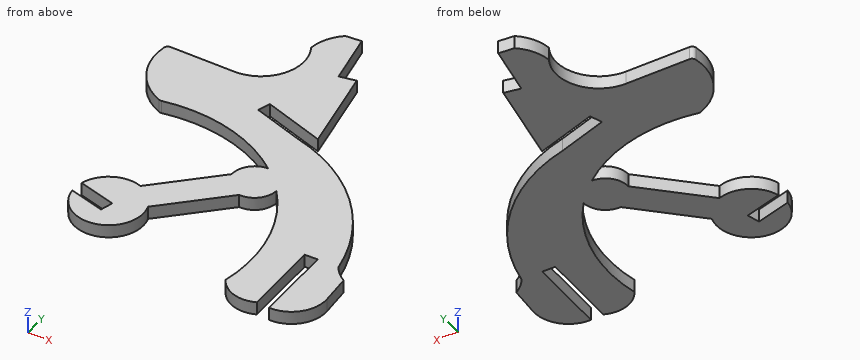
from build123d import *

# Parameters (mm, degrees)
BASE_EXTRUDE_DEPTH = 3


with BuildPart() as part:
    # Sketch1 → Base-Extrude (new body)
    with BuildSketch(Plane.XY):
        with BuildLine():
            Line((293.989820862, 734.197583092), (308.230093844, 729.586709902))
            Line((308.230093844, 729.586709902), (304.237578804, 749.960041406))
            Line((304.237578804, 749.960041406), (300.46187699, 749.205127022))
            Line((300.46187699, 749.205127022), (298.014696403, 761.444692703))
            Line((298.014696403, 761.444692703), (294.380010045, 761.126528526))
            ThreePointArc((294.380010045, 761.126528526), (291.873265467, 758.05762637), (290.76086587, 754.254404584))
            ThreePointArc((290.76086587, 754.254404584), (290.815065416, 744.34095117), (282.238682163, 739.368512483))
            Line((282.238682163, 739.368512483), (267.309755895, 739.368512483))
            ThreePointArc((267.309755895, 739.368512483), (266.660852695, 739.129383455), (266.322292677, 738.526361756))
            ThreePointArc((266.322292677, 738.526361756), (267.945922187, 729.535060668), (274.828113717, 723.525476008))
            ThreePointArc((274.828113717, 723.525476008), (275.107735881, 723.458131465), (275.394960471, 723.473160687))
            ThreePointArc((275.394960471, 723.473160687), (291.10707298, 723.128304911), (305.196249522, 716.165223024))
            ThreePointArc((305.196249522, 716.165223024), (301.525955586, 714.485747009), (300.152427977, 710.690339367))
            Line((300.152427977, 710.690339367), (287.135003329, 697.672914719))
            ThreePointArc((287.135003329, 697.672914719), (280.788235339, 697.185935894), (276.80604128, 692.2199775))
            Line((276.80604128, 692.2199775), (285.544339655, 689.832249216))
            Line((285.544339655, 689.832249216), (284.7535812, 686.938339057))
            Line((284.7535812, 686.938339057), (276.578441435, 689.172182037))
            ThreePointArc((276.578441435, 689.172182037), (286.308923255, 682.31315648), (292.084750798, 692.72316725))
            Line((292.084750798, 692.72316725), (305.102175446, 705.740591898))
            ThreePointArc((305.102175446, 705.740591898), (308.909028424, 707.124695347), (310.57796115, 710.815567264))
            ThreePointArc((310.57796115, 710.815567264), (317.662772954, 696.617074851), (318.003459515, 680.752785464))
            ThreePointArc((318.003459515, 680.752785464), (322.040475508, 677.537424223), (327.190781226, 677.869684733))
            Line((327.190781226, 677.869684733), (326.648810255, 696.184005937))
            Line((326.648810255, 696.184005937), (329.647496764, 696.272745292))
            Line((329.647496764, 696.272745292), (330.19785257, 677.675083141))
            ThreePointArc((330.19785257, 677.675083141), (336.159788883, 680.193967384), (338.280950791, 686.308714689))
            Line((338.280950791, 686.308714689), (337.692715429, 693.239584422))
            ThreePointArc((337.692715429, 693.239584422), (335.883457798, 694.612751583), (334.465786033, 696.387352382))
            ThreePointArc((334.465786033, 696.387352382), (324.143791375, 716.336225522), (304.697858302, 727.577079591))
            Line((304.697858302, 727.577079591), (293.065685578, 731.343473215))
            Line((293.065685578, 731.343473215), (293.989820862, 734.197583092))
        make_face()
    extrude(amount=BASE_EXTRUDE_DEPTH)


solid = part.part
The listing builds one solid part. Answer for the finished solid, in the listing's coordinates (mm). Coordinates: 2 decimals unless noted, no trailing zeros. Order: outer loops, then holes, each group sorted by start corner. A loop starts at its lowest first (then second) coordinate and runs counter-clockwise, first axis right, second up.
Q1. Consider line 1 (Y direction, x = 281, z = 2.85); line 2 (Y direction, x = 278, z = 0.4); line 3 (X direction, y = 693, z = 2.8). Determine where each line is inside the solid, lowest interval first.
Q2. A cutting plane is placed at B-B, the plane y = 753. Write down the section's boundary in (x, z), and give its area (3 significant figures).
Q3. A cutting plane is placed at C-C, the plane x = 315.5. Write down the section's boundary in (y, z).
Q4. Given P1, Ø1, axis at y = 749, z = 1.5, coming from the +X side, flat-ended and moving along its own axis, determine where the tip first touches the part or whether it passes through.
Answers follow:
1. line 1: y = 682.93 to 687.96, 691.07 to 697.29, 724.14 to 739.37
1. line 2: y = 685.48 to 688.78, 691.89 to 694.74, 723.89 to 739.37
1. line 3: x = 277.06 to 292.36, 318.36 to 326.74, 329.74 to 337.71
2. outline: (291.38, 0) - (299.7, 0) - (299.7, 3) - (291.38, 3) - close
2. area: 25.0 mm2
3. outline: (702.86, 0) - (723.19, 0) - (723.19, 3) - (702.86, 3) - close
4. P1: stops at x = 304.52
